Source: three-view drawing plus pictorial views. Frame: mm from the lowest corner of the part. A direction names the side the tool comes from. Coordinates: 2 decimals unless noted, no trailing zeros. Order: outer loops, then holes, each group sorted by start corner. A loop starts at its lowest first (then second) coordinate and runs counter-clockwise, first axis right, second up. Notation, with made-up numbers: (19.5, 48) -> (67.5, 48) arc R20 cw to (67.5, 64) -> close; hole circle Ø11 at (-17.75, 16). An arc over 180 degrees is marked (long way). Use one line per item in the form item = value. Start each with the question number.
1) Section query A-A on x = 8. Output: boundary loops of the cut face in (y, z).
2) Access query for the marked faces 1 and 2. Directions: +Z, -Z, +X, -X, +Y, -Y. A direction counts if a zero-diameter tool reaches every point of the face in a straight line with its end or side. Return the directions, or none.
3) Draft query along Y for the marked faces 3, 4, 5 and 6. Return one class per face: pulls with the +Y half, pulls with the -Y half, needs draft (parallel to the pull), parting line crosses it, or undercut.
4) Pin query (flat end, axial travel): pin 1 (3 mm diameter, centred on y = 7, z = 5, fed in from +X); pin 2 (1 mm diameter, centred on y = 9, z = 7.5, fed in from -X); pin 3 (5 mm diameter, centred on x = 2, y = 11.5, fed in from -Z). Return the tip coordinate at first contact, or that it passes through.
5) Section query C-C on y = 5.5. Output: boundary loops of the cut face in (x, z).
6) Section query B-B on z = 8. Output: boundary loops of the cut face in (x, y), then the cut area to 3 significant figures.
7) Ray query, line 1 along Y through (x, z) = (3, 13); line 2 along Z through (x, y) = (8, 10.25); line 3 along Z through (x, y) = (8, 4.25). Return the intervals inside material, ascending.
8) Section query D-D on z = 4.5. Output: boundary loops of the cut face in (x, y).
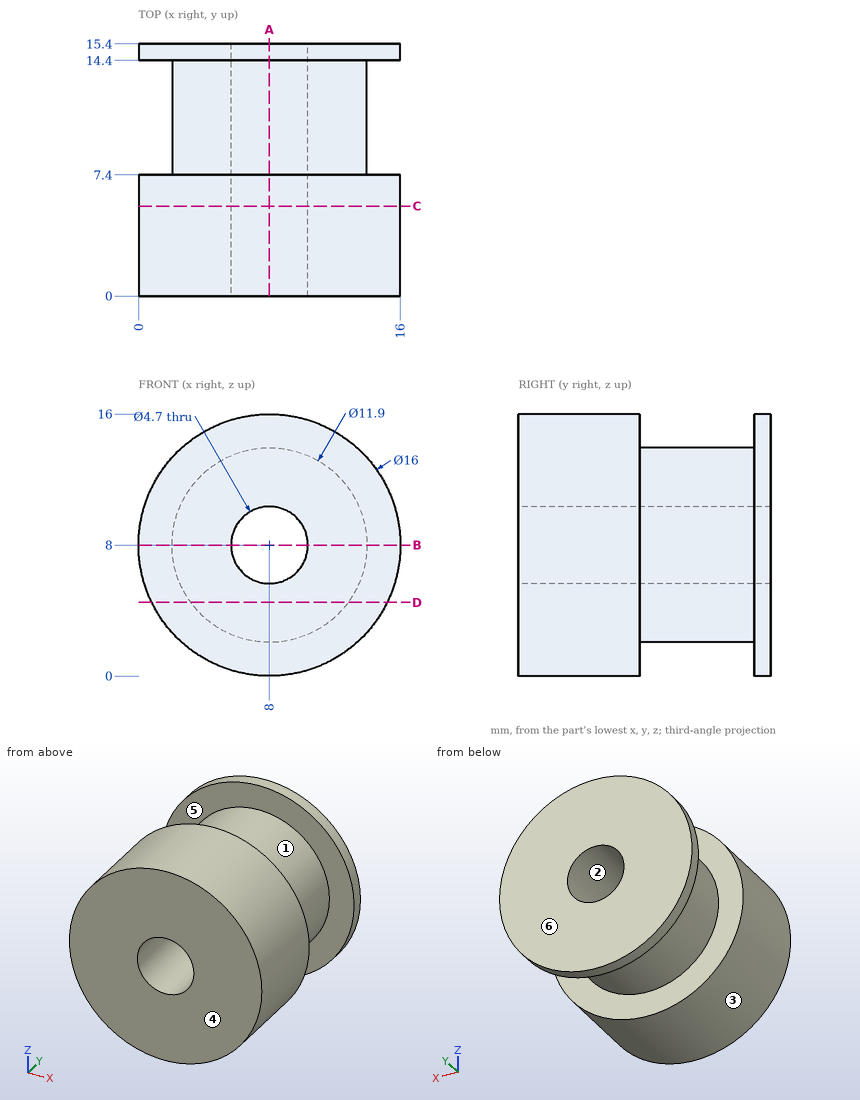
Answers below:
q1.outline = (0, 0) -> (7.4, 0) -> (7.4, 2.05) -> (14.4, 2.05) -> (14.4, 0) -> (15.4, 0) -> (15.4, 5.65) -> (0, 5.65) -> close; (0, 10.35) -> (15.4, 10.35) -> (15.4, 16) -> (14.4, 16) -> (14.4, 13.95) -> (7.4, 13.95) -> (7.4, 16) -> (0, 16) -> close
q2.face_1 = none
q2.face_2 = +Y, -Y
q3.face_3 = needs draft
q3.face_4 = pulls with the -Y half
q3.face_5 = undercut
q3.face_6 = pulls with the +Y half
q4.pin_1 = 15.86
q4.pin_2 = 2.05
q4.pin_3 = 3.19
q5.outline = circle Ø16 at (8, 8); hole circle Ø4.7 at (8, 8)
q6.outline = (0, 0) -> (5.65, 0) -> (5.65, 15.4) -> (0, 15.4) -> (0, 14.4) -> (2.05, 14.4) -> (2.05, 7.4) -> (0, 7.4) -> close; (10.35, 0) -> (16, 0) -> (16, 7.4) -> (13.95, 7.4) -> (13.95, 14.4) -> (16, 14.4) -> (16, 15.4) -> (10.35, 15.4) -> close
q6.area = 145 mm^2
q7.line_1 = 0 to 7.4, 14.4 to 15.4
q7.line_2 = 2.05 to 5.65, 10.35 to 13.95
q7.line_3 = 0 to 5.65, 10.35 to 16
q8.outline = (0.81, 0) -> (15.19, 0) -> (15.19, 7.4) -> (12.81, 7.4) -> (12.81, 14.4) -> (15.19, 14.4) -> (15.19, 15.4) -> (0.81, 15.4) -> (0.81, 14.4) -> (3.19, 14.4) -> (3.19, 7.4) -> (0.81, 7.4) -> close
